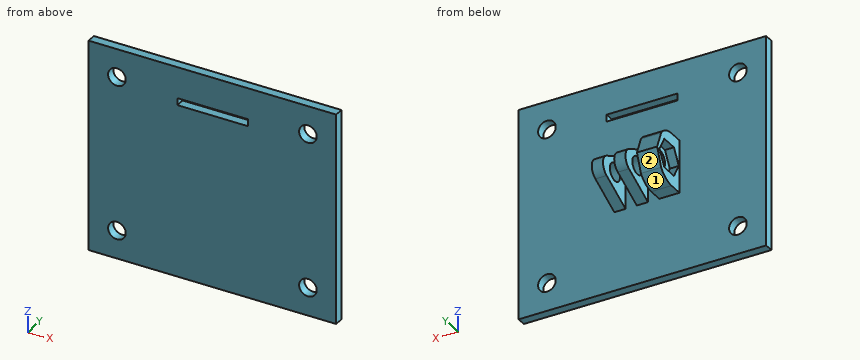
from build123d import *

# Parameters (mm, degrees)
SKETCH1_W                 = 70
SKETCH1_H                 = 60
SKETCH1_R                 = 2.5
BOSS_EXTRUDE1_DEPTH       = 2.54
SKETCH2_R                 = 1.651
BOSS_EXTRUDE2_DEPTH       = 7.9375
SKETCH3_W                 = 3.175
SKETCH3_H                 = 15
CUT_EXTRUDE1_DEPTH        = 15
FILLET1_R                 = 3.175
SKETCH6_W                 = 15
SKETCH6_H                 = 10.16
SKETCH6_R                 = 1.651
BOSS_EXTRUDE5_DEPTH       = 3.175
BOSS_EXTRUDE6_DEPTH       = 2.54
FILLET2_R                 = 6.35
F_5_0MM_DOWEL_HOLE1_D     = 5
F_5_0MM_DOWEL_HOLE1_DEPTH = 20
F_5_0MM_DOWEL_HOLE1_TIP   = 1.502151548
SKETCH10_W                = 20
SKETCH10_H                = 2
CUT_EXTRUDE2_DEPTH        = 10
BOSS_EXTRUDE8_DEPTH       = 2.54
CUT_EXTRUDE3_START        = -6.35
CUT_EXTRUDE3_DEPTH        = 6.35


with BuildPart() as part:
    # Sketch1 → Boss-Extrude1 (new body)
    with BuildSketch(Plane(origin=(0, 0, 0), x_dir=(1, 0, 0), z_dir=(0, 1, 0))):
        with Locations((0, 30)):
            Rectangle(SKETCH1_W, SKETCH1_H)
        with Locations(Location((-27, 52, 0), (0, 0, 270))):
            Circle(SKETCH1_R, mode=Mode.SUBTRACT)
        with Locations(Location((-27, 8, 0), (0, 0, 270))):
            Circle(SKETCH1_R, mode=Mode.SUBTRACT)
        with Locations(Location((27, 52, 0), (0, 0, 270))):
            Circle(SKETCH1_R, mode=Mode.SUBTRACT)
        with Locations(Location((27, 8, 0), (0, 0, 270))):
            Circle(SKETCH1_R, mode=Mode.SUBTRACT)
    extrude(amount=BOSS_EXTRUDE1_DEPTH)

    # Sketch2 → Boss-Extrude2 (add, symmetric)
    with BuildSketch(Plane(origin=(0, 0, 0), x_dir=(0, 0, -1), z_dir=(1, 0, 0))):
        Polygon((37.5, 2.54), (30, 17.54), (22.5, 2.54), align=None)
        with Locations((30, 7.62)):
            Circle(SKETCH2_R, mode=Mode.SUBTRACT)
    extrude(amount=BOSS_EXTRUDE2_DEPTH, both=True)

    # Sketch3 → Cut-Extrude1 (cut)
    with BuildSketch(Plane(origin=(0, 2.54, 0), x_dir=(1, 0, 0), z_dir=(0, 1, 0))):
        with Locations((-3.175, 30)):
            Rectangle(SKETCH3_W, SKETCH3_H)
        with Locations((3.175, 30)):
            Rectangle(SKETCH3_W, SKETCH3_H)
    extrude(amount=CUT_EXTRUDE1_DEPTH, mode=Mode.SUBTRACT)

    # Fillet1
    fillet1_edges = [part.edges().sort_by_distance(p)[0] for p in [
        (6.35, 17.54, -30),
        (-6.35, 17.54, -30),
        (0, 17.54, -30),
    ]]
    fillet(fillet1_edges, radius=FILLET1_R)

    # Sketch6 → Boss-Extrude5 (add)
    with BuildSketch(Plane.ZY.offset(7.9375)):
        with Locations((-30, 7.62)):
            Rectangle(SKETCH6_W, SKETCH6_H)
        with Locations((-30, 7.62)):
            Circle(SKETCH6_R, mode=Mode.SUBTRACT)
    extrude(amount=-BOSS_EXTRUDE5_DEPTH)

    # Sketch4 → Boss-Extrude6 (add)
    with BuildSketch(Plane.ZY.offset(7.9375)):
        Polygon((-37.5, 11.54), (-37.5, 2.54), (-22.5, 2.54), (-22.5, 11.54), (-28.589639166, 11.54), (-25.9, 9.987136104), (-25.9, 5.252863896), (-30, 2.885727793), (-34.1, 5.252863896), (-34.1, 9.987136104), (-31.410360834, 11.54), align=None)
    extrude(amount=BOSS_EXTRUDE6_DEPTH)

    # Fillet2
    # the kernel refuses this fillet: 6.35 mm, written as the material it takes off along each edge
    with BuildSketch(Plane(origin=(-23.580984977, 12.7, -22.5), x_dir=(0, 0, -1), z_dir=(1, 0, 0))) as fillet2_piece_1:
        with BuildLine():
            CenterArc((6.35, -6.257393991), FILLET2_R, 99.79714572, 80.202854281)
            Line((0, -6.257393991), (-0.127, -6.257393991))
            Line((-0.127, -6.257393991), (-0.127, 0))
            Line((-0.127, 0), (0, 0.127))
            ThreePointArc((0, 0.127), (2.634740701, 0.127), (5.247871029, 0.12514788))
            Line((5.247871029, 0.12514788), (5.269481401, 0))
        make_face()
    extrude(amount=34.461969954, mode=Mode.SUBTRACT)
    with BuildSketch(Plane(origin=(-23.580984977, 12.7, -37.5), x_dir=(0, 0, 1), z_dir=(1, 0, 0))) as fillet2_piece_2:
        with BuildLine():
            CenterArc((6.35, 6.257393991), FILLET2_R, 180, 80.202854281)
            Line((0, 6.257393991), (-0.127, 6.257393991))
            Line((-0.127, 6.257393991), (-0.127, 0))
            Line((-0.127, 0), (0, -0.127))
            ThreePointArc((0, -0.127), (2.634740701, -0.127), (5.247871029, -0.12514788))
            Line((5.247871029, -0.12514788), (5.269481401, 0))
        make_face()
    extrude(amount=34.461969954, mode=Mode.SUBTRACT)

    # Ø5.0mm Dowel Hole1
    with Locations(Plane(origin=(7.9375, 0, 0), x_dir=(0, 0, -1), z_dir=(1, 0, 0))):
        with Locations((29.751144641, 7.740920916)):
            Hole(F_5_0MM_DOWEL_HOLE1_D / 2, depth=F_5_0MM_DOWEL_HOLE1_DEPTH)
            with Locations((0, 0, -(F_5_0MM_DOWEL_HOLE1_DEPTH + F_5_0MM_DOWEL_HOLE1_TIP / 2))):  # 118° drill point
                Cone(0, F_5_0MM_DOWEL_HOLE1_D / 2, F_5_0MM_DOWEL_HOLE1_TIP, mode=Mode.SUBTRACT)

    # Sketch10 → Cut-Extrude2 (cut)
    with BuildSketch(Plane(origin=(0, 2.54, 0), x_dir=(1, 0, 0), z_dir=(0, 1, 0))):
        with Locations((0.117809829, 9.874502057)):
            Rectangle(SKETCH10_W, SKETCH10_H)
    extrude(amount=-CUT_EXTRUDE2_DEPTH, mode=Mode.SUBTRACT)

    # Sketch12 → Boss-Extrude8 (add)
    with BuildSketch(Plane.ZY.offset(7.9375)):
        Polygon((-31.410360834, 11.54), (-30, 12.354272207), (-28.589639166, 11.54), (-25.063302956, 11.54), (-30, 13.500615067), (-34.936697044, 11.54), align=None)
    extrude(amount=BOSS_EXTRUDE8_DEPTH)

    # Sketch13 → Cut-Extrude3 (cut)
    with BuildSketch(Plane.ZY.offset(7.9375).offset(CUT_EXTRUDE3_START)):
        with BuildLine():
            Line((-34.936697044, 11.54), (-30, 13.500615067))
            Line((-30, 13.500615067), (-25.063302956, 11.54))
            ThreePointArc((-25.063302956, 11.54), (-26.34823122, 12.279013549), (-27.769481401, 12.7))
            ThreePointArc((-27.769481401, 12.7), (-30, 13.615484171), (-32.230518599, 12.7))
            ThreePointArc((-32.230518599, 12.7), (-33.65176878, 12.279013549), (-34.936697044, 11.54))
        make_face()
    extrude(amount=CUT_EXTRUDE3_DEPTH, mode=Mode.SUBTRACT)


solid = part.part
Could you check a few things on this model? Use its own coordinates, in mm. Face numbers are marked on the shaded views. A direction names the side the tool comes from. Give positions to 0.01 mm unless a question says otherwise; leave off trailing zeros. Order: outer loops, then holes, each group sorted by start corner. A loop starts at its lowest first (then second) coordinate and runs counter-clockwise, first axis right, second up. Notation, with made-up numbers: (47, 81) - (67, 81) arc R15 cw to (67, 88) - close; hole circle Ø9 at (6.5, 66.5). An arc over 180 degrees is marked (long way). One line per item, written item: value. Start each with the question number.
1. For the marked faces 1 and 2, which set-ups out of +Z, -Z, +X, -X, +Y, -Y let a thin tool reach every point of the face, with its end or its side?
2. Imagine slicing it at D-D on z = -41. List the corners of the cut face in (x, y) for me, plus the area to 3 significant figures.
3. For P1, Ø3, axis at x = -7, y = 5, coming from the -Z side; P2, Ø6, axis at x = -27, z = -52, coming from the +Y side; P3, Ø4, axis at x = -25.5, y = 5.5, coming from the -Z side; P4, Ø1.3, axis at x = -9, y = 8.5, coming from the -Z side, each with a flat end and sliding along its axis, tell me the tip position at first contact or that it passes through.
4. Imagine slicing it at B-B on z = -6.5. List the corners of the cut face in (x, y) for me, plus the area to 3 significant figures.
5. If I drill on probe 1 along X at (y, z) = (1.05, -8); probe 2 along Z at (x, y) = (28, 1.75); probe 3 along Y at (x, z) = (-19, -13), over which ranges is the centre line in solid material (lowest first)?
6. Imagine slicing it at C-C on x = 4. List the corners of the cut face in (y, z) for me, plus the area to 3 significant figures.
7. Imagine slicing it at A-A on x = -27. List the corners of the cut face in (y, z) for me, plus the area to 3 significant figures.
Values:
1. face 1: -Z, +X, -X, +Y
1. face 2: -Z, -X, +Y
2. outline: (-35, 0) - (35, 0) - (35, 2.54) - (-35, 2.54) - close
2. area: 178 mm²
3. P1: z = -37.5
3. P2: y = 2.54
3. P3: through
3. P4: z = -37.34
4. outline: (-35, 0) - (-29, 0) - (-29, 2.54) - (-35, 2.54) - close; (-25, 0) - (25, 0) - (25, 2.54) - (-25, 2.54) - close; (29, 0) - (35, 0) - (35, 2.54) - (29, 2.54) - close
4. area: 157 mm²
5. probe 1: -35 to -29.5, -24.5 to 24.5, 29.5 to 35
5. probe 2: -60 to -54.29, -49.71 to -10.29, -5.71 to 0
5. probe 3: 0 to 2.54
6. outline: (0, -60) - (2.54, -60) - (2.54, -10.87) - (0, -10.87) - close; (0, -8.87) - (2.54, -8.87) - (2.54, 0) - (0, 0) - close
6. area: 147 mm²
7. outline: (0, -60) - (2.54, -60) - (2.54, -54.5) - (0, -54.5) - close; (0, -49.5) - (2.54, -49.5) - (2.54, -10.5) - (0, -10.5) - close; (0, -5.5) - (2.54, -5.5) - (2.54, 0) - (0, 0) - close
7. area: 127 mm²
